```python
from build123d import *

# Parameters (mm, degrees)
SKETCH1_R           = 40
BOSS_EXTRUDE1_DEPTH = 10
CUT_EXTRUDE1_REACH  = 59.446


with BuildPart() as part:
    # Sketch1 → Boss-Extrude1 (new body)
    with BuildSketch(Plane(origin=(0, 0, 0), x_dir=(1, 0, 0), z_dir=(0, 1, 0))):
        with Locations(Location((0, 0, 0), (0, 0, 270))):
            Circle(SKETCH1_R)
    extrude(amount=BOSS_EXTRUDE1_DEPTH)

    # Sketch2 → Cut-Extrude1 (cut, up to next)
    with BuildSketch(Plane(origin=(0, 10, 0), x_dir=(1, 0, 0), z_dir=(0, 1, 0)), mode=Mode.PRIVATE) as cut_extrude1_sk1:
        Polygon((11.238774325, 5.913221721), (0.497117057, 12.691874424), (-10.744197021, 6.778652704), (-11.243853833, -5.913221721), (-0.502196565, -12.691874424), (10.739117514, -6.778652704), align=None)
    cut_extrude1_tool1 = extrude(cut_extrude1_sk1.sketch, amount=-CUT_EXTRUDE1_REACH, mode=Mode.PRIVATE) & part.part
    # Sketch2 → Cut-Extrude1 (cut, up to next)
    with BuildSketch(Plane(origin=(0, 10, 0), x_dir=(1, 0, 0), z_dir=(0, 1, 0)), mode=Mode.PRIVATE) as cut_extrude1_sk2:
        with BuildLine():
            Line((34.543248704, -20.168390341), (28.580108202, -16.502199491))
            ThreePointArc((28.580108202, -16.502199491), (-2.229161984, -31.290031187), (-34.543248704, -20.168390341))
            ThreePointArc((-34.543248704, -20.168390341), (-19.915626859, -34.689592197), (0, -40))
            ThreePointArc((0, -40), (19.915626859, -34.689592197), (34.543248704, -20.168390341))
        make_face()
    cut_extrude1_tool2 = extrude(cut_extrude1_sk2.sketch, amount=-CUT_EXTRUDE1_REACH, mode=Mode.PRIVATE) & part.part
    # Sketch2 → Cut-Extrude1 (cut, up to next)
    with BuildSketch(Plane(origin=(0, 10, 0), x_dir=(1, 0, 0), z_dir=(0, 1, 0)), mode=Mode.PRIVATE) as cut_extrude1_sk3:
        with BuildLine():
            ThreePointArc((0, 33), (28.225744016, 13.532643941), (34.543248704, -20.168390341))
            ThreePointArc((34.543248704, -20.168390341), (34.689592197, 19.915626859), (0, 40))
            Line((0, 40), (0, 33))
        make_face()
    cut_extrude1_tool3 = extrude(cut_extrude1_sk3.sketch, amount=-CUT_EXTRUDE1_REACH, mode=Mode.PRIVATE) & part.part
    # Sketch2 → Cut-Extrude1 (cut, up to next)
    with BuildSketch(Plane(origin=(0, 10, 0), x_dir=(1, 0, 0), z_dir=(0, 1, 0)), mode=Mode.PRIVATE) as cut_extrude1_sk4:
        with BuildLine():
            ThreePointArc((0, 40), (-34.689592197, 19.915626859), (-34.543248704, -20.168390341))
            Line((-34.543248704, -20.168390341), (-28.580108202, -16.502199491))
            ThreePointArc((-28.580108202, -16.502199491), (-25.909016553, 17.626037907), (0, 40))
        make_face()
    cut_extrude1_tool4 = extrude(cut_extrude1_sk4.sketch, amount=-CUT_EXTRUDE1_REACH, mode=Mode.PRIVATE) & part.part
    add(cut_extrude1_tool1.solids().sort_by_distance((-0.00254, 10, 0))[0], mode=Mode.SUBTRACT)
    add(cut_extrude1_tool2.solids().sort_by_distance((5.104004, 10, 31.071916))[0], mode=Mode.SUBTRACT)
    add(cut_extrude1_tool3.solids().sort_by_distance((24.380546, 10, -19.814078))[0], mode=Mode.SUBTRACT)
    add(cut_extrude1_tool4.solids().sort_by_distance((-29.411799, 10, -11.104167))[0], mode=Mode.SUBTRACT)


solid = part.part
```
Work out the finished part from the listing and answer in its coordinate system (mm). A direction names the side the tool comes from. Coordinates: 2 decimals unless noted, no trailing zeros. Order: outer loops, then holes, each group sorted by start corner. A loop starts at its lowest first (then second) coordinate and runs counter-clockwise, first axis right, second up. Notation, with made-up numbers: (-32, 38) - (24, 38) arc R27 ccw to (24, 65) - close; hole circle Ø9 at (-30, 32.5). An arc over 180 degrees is marked (long way). Answer as a JSON object with one key per item and string values.
1. Find section C-C on x = -8.5. Determine the outline of the cut face in (y, z).
Output values:
{"outline": "(0, -36.14) - (10, -36.14) - (10, -7.96) - (0, -7.96) - close; (0, 7.64) - (10, 7.64) - (10, 31.22) - (0, 31.22) - close"}
2. The mould has two halves that part along X. Classify faces 6 (the face through (27.96, 5.07, -13.94)), 7 (the face through (1, 0, -13)), 8 (the face through (10.985, 5.07, 0.522)): +X half, -X half, draft (parallel to the pull), parting line (faces both ways), or undercut.
Output values:
{"face 6": "+X half", "face 7": "draft", "face 8": "undercut"}
3. Consider line 1 (X direction, y = 1, z = 20); line 2 (X direction, y = 3, z = -4); line 3 (Z direction, x = -7.5, y = 1.5). Determine where each line is inside the solid, lowest interval first.
Output values:
{"line 1": "x = -34.27 to 25.06, 34.27 to 34.58", "line 2": "x = -30.25 to -10.85, 11.16 to 32.92", "line 3": "z = -36.71 to -8.49, 8.28 to 31.29"}
4. Find section A-A on y = 8. Determine the outline of the cut face in (x, z), plus the area to 3 significant figures.
Output values:
{"outline": "(-34.54, 20.17) - (-28.58, 16.5) arc R45 ccw to (0, -40) - (0, -33) arc R45 ccw to (34.54, 20.17) - (28.58, 16.5) arc R45 ccw to start; hole (-11.24, 5.91) - (-10.74, -6.78) - (0.5, -12.69) - (11.24, -5.91) - (10.74, 6.78) - (-0.5, 12.69) - close", "area": "3,000 mm²"}
5. Find section B-B on z = -2.5. Determine the outline of the cut face in (x, y).
Output values:
{"outline": "(-30.45, 0) - (-10.91, 0) - (-10.91, 10) - (-30.45, 10) - close; (11.1, 0) - (33.42, 0) - (33.42, 10) - (11.1, 10) - close"}
6. Each of these flat-tipped pins is pushed along its axis until it touches: P1, Ø3, axis at x = -23.5, y = 2, coming from the -Z side; P2, Ø1.5, axis at x = -20, y = 5, coming from the -Z side; P3, Ø3.5, axis at y = 6.5, z = -35.5, coming from the +X side. Where does it stop, or does it pass through?
Output values:
{"P1": "stops at z = -23.98", "P2": "stops at z = -27.36", "P3": "stops at x = 0"}
7. A tool of negligible diameter and unlimited length cuts with its end or side. For faces 1 (the face through (1, 10, -13)), 2 (the face through (0, 5, -37)), 3 (the face through (31.6, 5.07, 18.36)), 4 (the face through (5.04, 5.07, 9.777)), 5 (the face through (-31.6, 5.07, 18.36)), from which of +Z, -Z, +X, -X, +Y, -Y can it reach the whole face along a straight path? Write none if from no direction.
Output values:
{"face 1": "+Z, -Z, +X, -X, +Y", "face 2": "-Z, +X, +Y, -Y", "face 3": "+Z, +Y, -Y", "face 4": "+Y, -Y", "face 5": "-X, +Y, -Y"}
8. Find section D-D on x = -22.5. Determine the outline of the cut face in (y, z), plus the area to 3 significant figures.
Output values:
{"outline": "(0, -23.29) - (10, -23.29) - (10, 27.75) - (0, 27.75) - close", "area": "510 mm²"}
